from build123d import *

# Parameters (mm, degrees)
SKETCH1_W           = 44.958
SKETCH1_H           = 304.8
BOSS_EXTRUDE1_DEPTH = 6.35
SKETCH2_W           = 6.35
SKETCH2_H           = 101.6
BOSS_EXTRUDE2_DEPTH = 6.35
SKETCH3_W           = 222.25
SKETCH3_H           = 6.35
BOSS_EXTRUDE3_DEPTH = 38.608
SKETCH7_W           = 327.022738736
SKETCH7_H           = 279.435650021
CUT_EXTRUDE1_DEPTH  = 45.958
SKETCH4_W           = 6.35
SKETCH4_H           = 6.35
SKETCH4_H_2         = 12.7
CUT_EXTRUDE2_DEPTH  = 6.35
SKETCH6_W           = 6.35
SKETCH6_H           = 16.933333333
SKETCH6_H_2         = 16.933333334
CUT_EXTRUDE3_DEPTH  = 7.35


with BuildPart() as part:
    # Sketch1 → Boss-Extrude1 (new body)
    with BuildSketch(Plane.XY):
        with Locations((-6.477, 3.048)):
            Rectangle(SKETCH1_W, SKETCH1_H)
        with BuildLine():
            Line((-3.302, 133.858), (-3.302, -143.002))
            Line((-3.302, -143.002), (3.302, -143.002))
            Line((3.302, -143.002), (3.302, 143.002))
            Line((3.302, 143.002), (-16.256, 143.002))
            Line((-16.256, 143.002), (-16.256, 136.398))
            Line((-16.256, 136.398), (-5.842, 136.398))
            ThreePointArc((-5.842, 136.398), (-4.045948776, 135.654051224), (-3.302, 133.858))
        make_face(mode=Mode.SUBTRACT)
    extrude(amount=BOSS_EXTRUDE1_DEPTH)

    # Sketch2 → Boss-Extrude2 (add)
    with BuildSketch(Plane(origin=(16.002, 0, 0), x_dir=(0, 0, -1), z_dir=(1, 0, 0))):
        Polygon((222.25, -60.452), (222.25, -47.752), (0, -47.752), (0, -149.352), (222.25, -149.352), (222.25, -136.652), (228.6, -136.652), (228.6, -119.718666667), (222.25, -119.718666667), (222.25, -107.018666667), (228.6, -107.018666667), (228.6, -90.085333333), (222.25, -90.085333333), (222.25, -77.385333333), (228.6, -77.385333333), (228.6, -60.452), align=None)
        with BuildLine():
            ThreePointArc((11.4, -116.592), (9.9, -118.092), (8.4, -116.592))
            Line((8.4, -116.592), (8.4, -111.512))
            ThreePointArc((8.4, -111.512), (9.9, -110.012), (11.4, -111.512))
            Line((11.4, -111.512), (11.4, -116.592))
        make_face(mode=Mode.SUBTRACT)
        with BuildLine():
            Line((42.4, -111.512), (42.4, -116.592))
            ThreePointArc((42.4, -116.592), (40.9, -118.092), (39.4, -116.592))
            Line((39.4, -116.592), (39.4, -111.512))
            ThreePointArc((39.4, -111.512), (40.9, -110.012), (42.4, -111.512))
        make_face(mode=Mode.SUBTRACT)
        with BuildLine():
            ThreePointArc((36.4, -101.092), (25.4, -112.092), (14.4, -101.092))
            Line((14.4, -101.092), (14.4, -96.012))
            ThreePointArc((14.4, -96.012), (25.4, -85.012), (36.4, -96.012))
            Line((36.4, -96.012), (36.4, -101.092))
        make_face(mode=Mode.SUBTRACT)
        with BuildLine():
            ThreePointArc((11.4, -85.592), (9.9, -87.092), (8.4, -85.592))
            Line((8.4, -85.592), (8.4, -80.512))
            ThreePointArc((8.4, -80.512), (9.9, -79.012), (11.4, -80.512))
            Line((11.4, -80.512), (11.4, -85.592))
        make_face(mode=Mode.SUBTRACT)
        with BuildLine():
            ThreePointArc((42.4, -85.592), (40.9, -87.092), (39.4, -85.592))
            Line((39.4, -85.592), (39.4, -80.512))
            ThreePointArc((39.4, -80.512), (40.9, -79.012), (42.4, -80.512))
            Line((42.4, -80.512), (42.4, -85.592))
        make_face(mode=Mode.SUBTRACT)
        with Locations((-3.175, -98.552)):
            Rectangle(SKETCH2_W, SKETCH2_H)
    extrude(amount=-BOSS_EXTRUDE2_DEPTH)

    # Sketch3 → Boss-Extrude3 (add)
    with BuildSketch(Plane.ZY.offset(-9.652)):
        with Locations((-111.125, -146.177)):
            Rectangle(SKETCH3_W, SKETCH3_H)
    extrude(amount=BOSS_EXTRUDE3_DEPTH)

    # Sketch7 → Cut-Extrude1 (cut, through all)
    with BuildSketch(Plane(origin=(16.002, 0, 0), x_dir=(0, 0, -1), z_dir=(1, 0, 0))):
        with Locations((163.511369368, -148.348068682)):
            Rectangle(SKETCH7_W, SKETCH7_H)
    extrude(amount=-CUT_EXTRUDE1_DEPTH, mode=Mode.SUBTRACT)

    # Sketch4 → Cut-Extrude2 (cut)
    with BuildSketch(Plane.XZ.offset(149.352)):
        with Locations((-12.954, 3.175)):
            Rectangle(SKETCH4_W, SKETCH4_H)
        with Locations((12.827, 3.175)):
            Rectangle(SKETCH4_W, SKETCH4_H)
        with Locations((-25.781, 3.175)):
            Rectangle(SKETCH4_W, SKETCH4_H)
        with Locations((12.827, -134.9375)):
            Rectangle(SKETCH4_W, SKETCH4_H_2)
        with Locations((12.827, -53.975)):
            Rectangle(SKETCH4_W, SKETCH4_H_2)
        with Locations((12.827, -161.925)):
            Rectangle(SKETCH4_W, SKETCH4_H_2)
    extrude(amount=-CUT_EXTRUDE2_DEPTH, mode=Mode.SUBTRACT)

    # Sketch6 → Cut-Extrude3 (cut, through all)
    with BuildSketch(Plane.XY.offset(6.35)):
        with Locations((12.827, -68.918666667)):
            Rectangle(SKETCH6_W, SKETCH6_H)
        with Locations((12.827, -98.552)):
            Rectangle(SKETCH6_W, SKETCH6_H_2)
        with Locations((12.827, -128.185333334)):
            Rectangle(SKETCH6_W, SKETCH6_H)
    extrude(amount=-CUT_EXTRUDE3_DEPTH, mode=Mode.SUBTRACT)


solid = part.part
CAD build for the part. Positions are in the model's coordinates, mm. A direction names the side the tool comes from. Round coordinates to 2 decimals unless told otherwise and drop trailing zeros. Write each loop counter-clockwise with the first axis right and the second up, starting at its lowest first coordinate (ties: lowest second). Pieces come first, ordered by that corner, then holes. Notation, with made-up numbers: (13, 4.5) -> (23, 4.5) arc R14 cw to (23, 18.5) -> close; hole circle Ø1 at (0.25, -2). An arc over 180 degrees is marked (long way). Answer as a JSON object with one key per item and string values.
(1) Two-plate mould, pull along X, no slides. Class faces 6 (the face through (-28.956, 8, 3)), 7 (the face through (-19, -149.352, 3)), 8 (the face through (-11, 136.398, 3)): +X half, -X half, draft (parallel to the pull), parting line (faces both ways), or undercut.
Reported:
{"face 6": "-X half", "face 7": "draft", "face 8": "undercut"}
(2) Pin check, flat tips, straight feed: P1, Ø3, axis at x = 12, z = 3.5, coming from the -Y side; P2, Ø6, axis at x = 11.5, y = -66.5, coming from the -Z side; P3, Ø1.9, axis at y = -100, z = 2, coming from the +X side; P4, Ø1.9, axis at y = -147, z = 3.5, coming from the -X side. Stop position of each tip, or through.
Reported:
{"P1": "stops at y = -143", "P2": "stops at z = 0", "P3": "stops at x = 9.65", "P4": "stops at x = -22.61"}
(3) Probe probe 1 along X at (y, z) = (84, 1.5); probe 2 along X at (y, z) = (-74.5, 2.25); probe 3 along Y at (x, z) = (-14, 5.5). List the from-to ranges inside material, lowest first. Write a range as [from, to].
Reported:
{"probe 1": "x = [-28.96, -3.3], [3.3, 16]", "probe 2": "x = [-28.96, -3.3], [3.3, 9.65]", "probe 3": "y = [-143, 136.4], [143, 155.45]"}
(4) Band-saw the part on B-B, the plane y = -112. List the corners of the cut face in (x, z).
Reported:
{"outline": "(-28.96, 0) -> (-3.3, 0) -> (-3.3, 6.35) -> (-28.96, 6.35) -> close; (3.3, 0) -> (16, 0) -> (16, 6.35) -> (3.3, 6.35) -> close"}
(5) Which spindle directions (+Z, -Z, +X, -X, +Y, -Y) get a long thin tool onto all of the face, cutting with end or side? Do faces 1 (the face through (-13, -143.002, 3)), 2 (the face through (-26, -143.002, 3)), 3 (the face through (9.652, -146, 3)), 4 (the face through (-16.256, 140, 3)), 5 (the face through (13, -119.719, 3)). Say none if no direction does.
Reported:
{"face 1": "+Z, -Z, -Y", "face 2": "+Z, -Z, -X, -Y", "face 3": "+Z, -Z, +X, -Y", "face 4": "+Z, -Z", "face 5": "+Z, -Z, +X"}
(6) Band-saw the part on C-C, the plane x = -13.5. List the corners of the cut face in (y, z).
Reported:
{"outline": "(-143, 0) -> (136.4, 0) -> (136.4, 6.35) -> (-143, 6.35) -> close; (143, 0) -> (155.45, 0) -> (155.45, 6.35) -> (143, 6.35) -> close"}
